Can you work these out from the model? Positions are in its coordinate system, mm. A direction names the side the tool comes from. Coordinates: 2 decimals unless noted, no trailing zeros. Order: outer loops, then holes, each group sorted by start corner. A loop starts at its lowest first (then second) coordinate and runs counter-clockwise, first axis right, second up. Notation, with made-up numbers: M 70.5,84.25 L 107.5,84.25 A30 ccw 107.5,119.25 Z; hole C 54.25,81 d7. An arc over 180 degrees is marked long. Answer as a JSON object with one key per item and string values.
from build123d import *

# Parameters (mm, degrees)
F1_DEPTH = 20
F2_W     = 6.5510021523
F2_H     = 6.1886049807
F3_DEPTH = 5
F4_R     = 5.6777996294
F4_R_2   = 2.4237453519
F5_DEPTH = 10


with BuildPart() as f1:
    # F0 (on Right) → F1 (new body)
    with BuildSketch(Plane.YZ):
        Polygon((-46.2598241866, -13.305501081), (-50.5918487906, -13.305501081), (-50.5918487906, -18.2563848794), (-40.6900793314, -18.2563848794), (-40.6900793314, 10.8300596476), (-30.7883117348, 10.8300596476), (-30.7883117348, -18.2563848794), (-17.7922397852, -18.2563848794), (-17.7922397852, -12.0677798986), (-23.9808466285, -12.0677798986), (-23.9808466285, 18.8752468675), (-46.2598241866, 18.8752468675), align=None)
    extrude(amount=F1_DEPTH)

    # F2 (on face) → F3 (cut)
    with BuildSketch(Plane(origin=(0, -17.7922397852, 0), x_dir=(-1, 0, 0), z_dir=(0, 1, 0))):
        with Locations((-9.8014348187, -15.162082389)):
            Rectangle(F2_W, F2_H)
    extrude(amount=-F3_DEPTH, mode=Mode.SUBTRACT)

    # F4 (on face) → F5 (join)
    with BuildSketch(Plane(origin=(0, -23.9808466285, 0), x_dir=(-1, 0, 0), z_dir=(0, 1, 0))):
        with Locations((-13.9073636383, 8.8768014684)):
            Circle(F4_R)
        with Locations((-13.9073636383, 8.8768014684)):
            Circle(F4_R_2, mode=Mode.SUBTRACT)
    extrude(amount=F5_DEPTH)


solid = f1.part
Item 1: I want a section at B-B, the plane y = -23.5. Write out the boundary of the cut face in (x, z).
Answers follow:
{"outline": "M 0,-18.26 L 20,-18.26 L 20,-12.07 L 0,-12.07 Z; C 13.91,8.88 d11.36; hole C 13.91,8.88 d4.85"}
Item 2: I want a section at C-C, the plane x = 4.75. Write out the boundary of the cut face in (y, z), plus the area to 3 significant figures.
Answers follow:
{"outline": "M -50.59,-18.26 L -40.69,-18.26 L -40.69,10.83 L -30.79,10.83 L -30.79,-18.26 L -17.79,-18.26 L -17.79,-12.07 L -23.98,-12.07 L -23.98,18.88 L -46.26,18.88 L -46.26,-13.31 L -50.59,-13.31 Z", "area": "599 mm^2"}
Item 3: I'm going to push flat-ended pins straight in: pin 1 (4.5 mm diameter, centred on x = 13.91, z = 8.88, fed in from -Y); pin 2 (5 mm diameter, centred on x = 10.5, z = -15.5, fed in from +Y); pin 3 (2.5 mm diameter, centred on x = 14, z = 9, fed in from +Y); pin 4 (6 mm diameter, centred on y = -34, z = -9, fed in from +X). Where does each tip first touch, or does it pass through?
Answers follow:
{"pin 1": "stops at y = -46.26", "pin 2": "stops at y = -22.79", "pin 3": "stops at y = -23.98", "pin 4": "passes through"}
Item 4: If we mould it in two halves opening along Z, with no side actions, what happens to faces 1 (the flat face through (10, -23.981, 3)), 2 (the flat face through (10, -46.26, 3)), 3 (the flat face through (10, -24, -18.256)), 4 (the cylindrical face through (8.663, -19.051, 6.702))? For each: pulls with the +Z half, pulls with the -Z half, needs draft (parallel to the pull), parting line crosses it, or undercut.
Answers follow:
{"face 1": "undercut", "face 2": "needs draft", "face 3": "pulls with the -Z half", "face 4": "undercut"}
Item 5: Please list where these lines run through material, in increasing order: line 1 (Y direction, x = 16, z = -10); line 2 (Z direction, x = 14, y = -18); line 3 (Y direction, x = 9.5, z = 6).
Answers follow:
{"line 1": "y = -46.26 to -40.69, -30.79 to -23.98", "line 2": "z = -18.26 to -12.07, 3.2 to 6.45, 11.3 to 14.55", "line 3": "y = -46.26 to -40.69, -30.79 to -13.98"}
Item 6: Which directions (+Z, -Z, +X, -X, +Y, -Y) give clear straight access to the entire face, cutting with the end or side of a thin tool? Please do faces 5 (the flat face through (10, -30.788, -4)), 6 (the flat face through (13.077, -20, -15)), 7 (the cylindrical face through (15.83, -19.05, 7.4)).
Answers follow:
{"face 5": "-Z, +X, -X", "face 6": "-Z, +Y", "face 7": "+Y"}
Item 7: I want a section at A-A, the plane z = -7. Write out the boundary of the cut face in (x, y), plus the area to 3 significant figures.
Answers follow:
{"outline": "M 0,-46.26 L 20,-46.26 L 20,-40.69 L 0,-40.69 Z; M 0,-30.79 L 20,-30.79 L 20,-23.98 L 0,-23.98 Z", "area": "248 mm^2"}
Item 8: I want a section at D-D, the plane z = 14. Write out the boundary of the cut face in (x, y).
Answers follow:
{"outline": "M 0,-46.26 L 20,-46.26 L 20,-23.98 L 16.35,-23.98 L 16.35,-13.98 L 11.46,-13.98 L 11.46,-23.98 L 0,-23.98 Z"}
